Design review of the part shown in the three views and the two pictorial views. Dimensions are in mm from the part's minimum x, y and z. A direction names the side the tool comes from. Coordinates: 2 decimals unless noted, no trailing zeros. Write each loop counter-clockwise with the first axis right and the second up, starting at its lowest first coordinate (ties: lowest second). Pieces come first, ordered by that corner, then holes. Notation, with made-up numbers: (87, 64.25) -> (141, 64.25) arc R24 ccw to (141, 96.25) -> close; hole circle Ø5 at (47.5, 87). An arc over 180 degrees is marked (long way). Answer in a Markdown table with one row per item. Add a question column.
Item 1: Take a section at B-B, the plane x = 30. Write out the cut boundary in (y, z).
Item 2: For the marked faces 5, 6, 7 and 8, list the 3-axis set-ups (+Z, -Z, +X, -X, +Y, -Y) from which the entire face can be reached by the end or side of a thin tool; tool diameter is ignored.
Item 3: To check wall thickness, follow line 1 (X direction, y = 23, z = 7.5); line 2 (Y direction, x = 36, z = 5.25); line 3 (Z direction, x = 22, y = 10.25). State the ranges of each line that lie inside material, in increasing order.
Item 4: Clearance check with flat-ended pins moving along their axes: P1, Ø2, axis at x = 13, z = 11, coming from the +Y side; P2, Ø1.5, axis at x = 6, y = 5.5, coming from the +Z side; P3, Ø6.5, axis at x = 33, z = 10, coming from the +Y side. State where each tip first meets the part, or that it passes through.
Item 5: Take a section at D-D, the plane z = 1. Write out the cut boundary in (x, y).
Item 6: Draft analysis for pull direction Y (two halves, no side actions). For the marked faces 1, 2, 3 and 4, state which applies: released by +Y, released by -Y, zero draft, split by the parting line, or undercut.
Item 7: Take a section at C-C, the plane y = 10.5. Write out the cut boundary in (x, z).
Item 8: Take a section at A-A, the plane z = 6. Write out the cut boundary in (x, y), and give its area (3 significant figures).
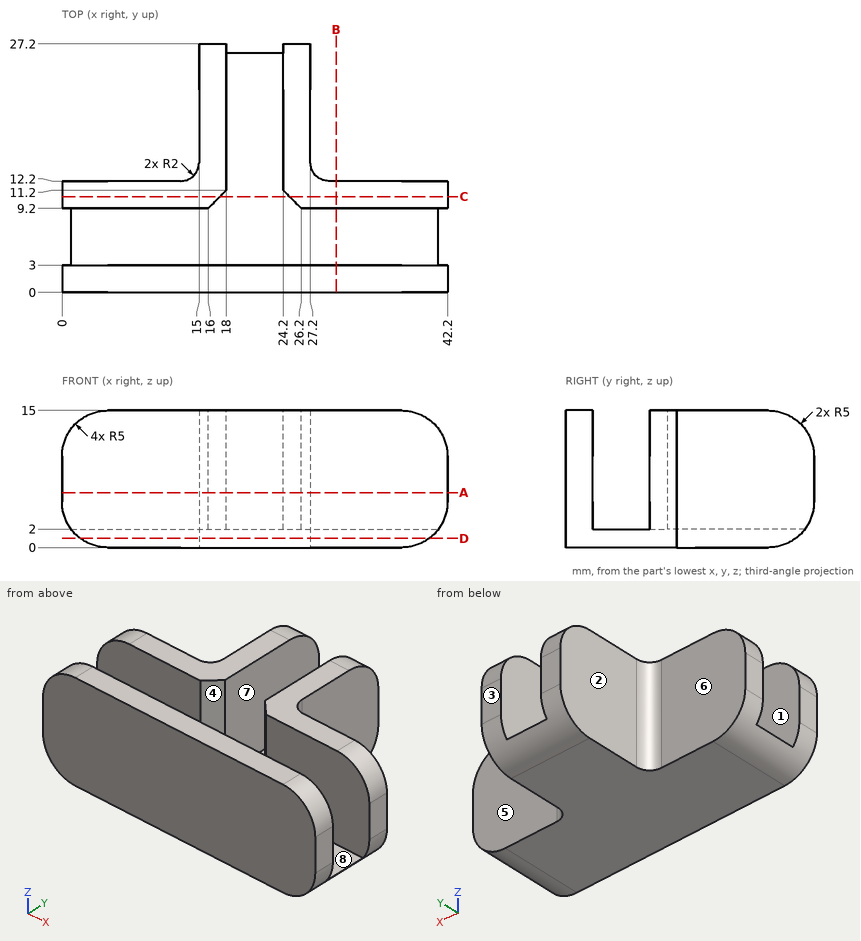
Answers:
| question | item | result |
|---|---|---|
| 1 | outline | (0, 0) -> (12.2, 0) -> (12.2, 15) -> (9.2, 15) -> (9.2, 2) -> (3, 2) -> (3, 15) -> (0, 15) -> close |
| 2 | face 5 | +Z, -Z, +X, +Y |
| 2 | face 6 | +Z, -Z, -X, +Y |
| 2 | face 7 | +Z, +Y |
| 2 | face 8 | +Z |
| 3 | line 1 | x = 15 to 18, 24.2 to 27.2 |
| 3 | line 2 | y = 0 to 3, 9.2 to 12.2 |
| 3 | line 3 | z = 0 to 2 |
| 4 | P1 | stops at y = 12.47 |
| 4 | P2 | stops at z = 2 |
| 4 | P3 | stops at y = 12.2 |
| 5 | outline | (2, 0) -> (40.2, 0) -> (40.2, 12.2) -> (29.2, 12.2) arc R2 cw to (27.2, 14.2) -> (27.2, 25.2) -> (15, 25.2) -> (15, 14.2) arc R2 cw to (13, 12.2) -> (2, 12.2) -> close |
| 6 | face 1 | undercut |
| 6 | face 2 | zero draft |
| 6 | face 3 | released by +Y |
| 6 | face 4 | undercut |
| 7 | outline | (0, 5) arc R5 ccw to (5, 0) -> (37.2, 0) arc R5 ccw to (42.2, 5) -> (42.2, 10) arc R5 ccw to (37.2, 15) -> (24.9, 15) -> (24.9, 2) -> (17.3, 2) -> (17.3, 15) -> (5, 15) arc R5 ccw to (0, 10) -> close |
| 8 | outline | (0, 0) -> (42.2, 0) -> (42.2, 3) -> (0, 3) -> close; (0, 9.2) -> (16, 9.2) -> (18, 11.2) -> (18, 27.2) -> (15, 27.2) -> (15, 14.2) arc R2 cw to (13, 12.2) -> (0, 12.2) -> close; (24.2, 11.2) -> (26.2, 9.2) -> (42.2, 9.2) -> (42.2, 12.2) -> (29.2, 12.2) arc R2 cw to (27.2, 14.2) -> (27.2, 27.2) -> (24.2, 27.2) -> close |
| 8 | area | 322 mm^2 |
